Here's how the part is built. I have some questions about the finished solid (model axes, mm). Face numbers are marked on the shaded views. A direction names the side the tool comes from. Give positions to 0.01 mm unless a question says otherwise; leave off trailing zeros. Write each loop counter-clockwise with the first axis right and the second up, starting at its lowest first coordinate (ties: lowest second). Pieces come first, ordered by that corner, then holes. Notation, with made-up numbers: (-23.5, -20) -> (35.5, -20) arc R17 ccw to (35.5, 1) -> close; hole circle Ø11 at (43, 81). An arc over 180 degrees is marked (long way). Use CSV: the item, a comma, the result in double quotes. Start each with the question number.
(1) Which directions (+Z, -Z, +X, -X, +Y, -Y) give clear straight access to the entire face, cutting with the end or side of a thin tool? Please do the marked faces 1 and 2.
(2) Suppose I cut it at D-D on y = 117.5. List the corners of the cut face in (x, z) for me, plus the area to 3 significant figures.
(3) Suppose I cut it at C-C on y = 185.5. List the corners of the cut face in (x, z) for me, plus the area to 3 significant figures.
(4) I need wall thicknesses on L1, parallel to Z at x = -0.5, y = 185; L2, parallel to X at y = 29, z = 18; L3, parallel to Z at x = 15, y = 109.5. Which ranges of each line are inside material? Lowest first, please. Write a range as [from, to].
(5) For pin 1 Ø8 at (y, z) = (28.5, -3.5) entering from +X; pin 2 Ø12 at (x, y) = (16.5, 99) entering from +Z; pin 3 Ø1.5 at (x, y) = (-12, 171) entering from +Z, each with a flat end and sliding along its axis, tell me the tip position at first contact or that it passes through.
from build123d import *

# Parameters (mm, degrees)
ESQUISSE1_R         = 37.5
EXTRUSION1_DEPTH    = 200
ESQUISSE2_OUTSIDE_W = 122.276
ESQUISSE2_OUTSIDE_H = 122.276
ESQUISSE2_OUTSIDE_R = 15
EXTRUSION2_DEPTH    = 20
CHANFREIN1_SIZE     = 22.5


with BuildPart() as part:
    # Esquisse1 → Extrusion1 (new body)
    with BuildSketch(Plane(origin=(0, 0, 0), x_dir=(1, 0, 0), z_dir=(0, 1, 0))):
        with Locations(Location((0, 0, 0), (0, 0, 270))):
            Circle(ESQUISSE1_R)
    extrude(amount=EXTRUSION1_DEPTH)

    # Esquisse2 outside → Extrusion2 (cut)
    with BuildSketch(Plane(origin=(0, 200, 0), x_dir=(1, 0, 0), z_dir=(0, 1, 0))):
        Rectangle(ESQUISSE2_OUTSIDE_W, ESQUISSE2_OUTSIDE_H)
        with Locations(Location((0, 0, 0), (0, 0, 270))):
            Circle(ESQUISSE2_OUTSIDE_R, mode=Mode.SUBTRACT)
    extrude(amount=-EXTRUSION2_DEPTH, mode=Mode.SUBTRACT)

    # Chanfrein1
    chanfrein1_edges = [part.edges().sort_by_distance(p)[0] for p in [
        (0, 180, -37.5),
    ]]
    chamfer(chanfrein1_edges, length=CHANFREIN1_SIZE - 0.0001)  # a hair under: the kernel refuses the full size


solid = part.part
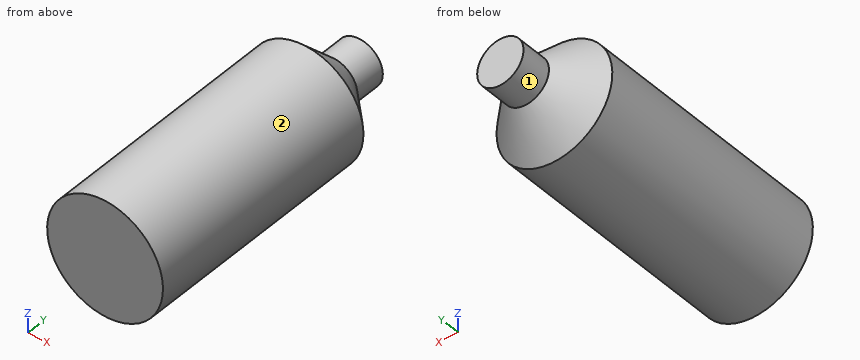
Geometry says:
1,face 1,"+Y"
1,face 2,"+Y, -Y"
2,outline,"circle Ø75 at (0, 0)"
2,area,"4,420 mm²"
3,outline,"circle Ø30 at (0, 0)"
3,area,"707 mm²"
4,L1,"[-14.99, 14.99]"
4,L2,"[-32.9, 32.9]"
4,L3,"[-34.37, 34.37]"
5,pin 1,"x = 37.5"
5,pin 2,"z = 36"
5,pin 3,"z = 21.74"
